from build123d import *

# Parameters (mm, degrees)
SKETCH1_R               = 43.5
SKETCH1_R_2             = 33.5
BOSS_EXTRUDE1_DEPTH     = 3
SKETCH3_R               = 2.025
CUT_EXTRUDE2_DEPTH      = 62.591395503
CIRPATTERN1_COUNT       = 12
CUT_EXTRUDE1_DEPTH      = 62.591395503
BOSS_EXTRUDE2_DEPTH     = 3
CUT_EXTRUDE_THIN1_DEPTH = 3
FILLET1_R               = 1.2
FILLET2_R               = 5
SKETCH6_R               = 2.525
CUT_EXTRUDE3_DEPTH      = 108.998410492
MIRROR4_OUTLINE_R       = 2.525
MIRROR4_DEPTH           = 3


# Read off the part's stored shape, not the designer's step: Mirror4
with BuildPart() as part:
    # Sketch1 → Boss-Extrude1 (new body)
    with BuildSketch(Plane(origin=(0, 0, 0), x_dir=(1, 0, 0), z_dir=(0, 1, 0))):
        with Locations(Location((0, 0, 0), (0, 0, 270))):
            Circle(SKETCH1_R)
        with Locations(Location((0, 0, 0), (0, 0, 270))):
            Circle(SKETCH1_R_2, mode=Mode.SUBTRACT)
    extrude(amount=BOSS_EXTRUDE1_DEPTH)

    # Sketch3 → Cut-Extrude2 (cut, symmetric)
    with BuildSketch(Plane(origin=(0, 3, 0), x_dir=(1, 0, 0), z_dir=(0, 1, 0))):
        with Locations(Location((-38, 0, 0), (0, 0, 270))):
            Circle(SKETCH3_R)
    cut_extrude2 = extrude(amount=CUT_EXTRUDE2_DEPTH, both=True, mode=Mode.SUBTRACT)

    # CirPattern1: Cut-Extrude2 ×12 about axis
    cirpattern1_axis = Axis((0, 0, 0), (0, 1, 0))
    for i in range(1, CIRPATTERN1_COUNT):
        add(cut_extrude2.rotate(cirpattern1_axis, i * 360 / CIRPATTERN1_COUNT), mode=Mode.SUBTRACT)

    # Sketch2 → Cut-Extrude1 (cut, symmetric)
    with BuildSketch(Plane(origin=(0, 3, 0), x_dir=(1, 0, 0), z_dir=(0, 1, 0))):
        with BuildLine():
            Line((0, 0), (43.5, 0))
            ThreePointArc((43.5, 0), (24.950574981, -35.633113927), (-14.877876235, -40.876629004))
            Line((-14.877876235, -40.876629004), (0, 0))
        make_face()
    cut_extrude1 = extrude(amount=CUT_EXTRUDE1_DEPTH, both=True, mode=Mode.SUBTRACT)

    # Mirror1: Cut-Extrude1 across plane
    add(cut_extrude1.mirror(Plane.XY), mode=Mode.SUBTRACT)

    # Sketch4 → Boss-Extrude2 (add)
    with BuildSketch(Plane(origin=(0, 0, 0), x_dir=(1, 0, 0), z_dir=(0, 1, 0))):
        with BuildLine():
            ThreePointArc((-33.322933276, -27.961261021), (-36.687527893, -23.372532963), (-39.424388736, -18.383894386))
            Line((-39.424388736, -18.383894386), (-57.550544477, -26.836259621))
            Line((-57.550544477, -26.836259621), (-76.583008005, -35.711243117))
            ThreePointArc((-76.583008005, -35.711243117), (-57.087372544, -62.29993496), (-28.900702111, -79.404026456))
            Line((-28.900702111, -79.404026456), (-21.718279101, -59.67048142))
            ThreePointArc((-21.718279101, -59.67048142), (-36.422103708, -52.016154812), (-48.643822138, -40.817013215))
            Line((-48.643822138, -40.817013215), (-33.322933276, -27.961261021))
        make_face()
    extrude(amount=BOSS_EXTRUDE2_DEPTH)

    # Sketch5 → Cut-Extrude-Thin1 (cut)
    with BuildSketch(Plane(origin=(0, 3, 0), x_dir=(1, 0, 0), z_dir=(0, 1, 0))):
        with BuildLine():
            ThreePointArc((-55.318354903, -43.219435568), (-42.735052316, -55.693404488), (-27.42932522, -64.619440712))
            Line((-27.42932522, -64.619440712), (-26.491570512, -62.410229064))
            ThreePointArc((-26.491570512, -62.410229064), (-41.274024887, -53.789356472), (-53.427129095, -41.741848027))
            Line((-53.427129095, -41.741848027), (-55.318354903, -43.219435568))
        make_face()
        with BuildLine():
            ThreePointArc((-62.804457062, -49.068219583), (-48.518285892, -63.230261221), (-31.141270941, -73.36423682))
            Line((-31.141270941, -73.36423682), (-30.203516232, -71.155025172))
            ThreePointArc((-30.203516232, -71.155025172), (-47.057258462, -61.326213205), (-60.913231254, -47.590632043))
            Line((-60.913231254, -47.590632043), (-62.804457062, -49.068219583))
        make_face()
    extrude(amount=-CUT_EXTRUDE_THIN1_DEPTH, mode=Mode.SUBTRACT)

    # Fillet1
    fillet1_edges = [part.edges().sort_by_distance(p)[0] for p in [
        (-55.318354903, 1.5, 43.219435568),
        (-62.804457062, 1.5, 49.068219583),
        (-53.427129095, 1.5, 41.741848027),
        (-60.913231254, 1.5, 47.590632043),
        (-26.491570512, 1.5, 62.410229064),
        (-30.203516232, 1.5, 71.155025172),
        (-27.42932522, 1.5, 64.619440712),
        (-31.141270941, 1.5, 73.36423682),
    ]]
    fillet(fillet1_edges, radius=FILLET1_R - 0.0001)  # a hair under: the kernel refuses the full size

    # Fillet2
    fillet2_edges = [part.edges().sort_by_distance(p)[0] for p in [
        (-14.877876235, 1.5, -40.876629004),
        (-11.457674801, 1.5, -31.479702796),
        (-11.457674801, 1.5, 31.479702796),
        (-14.877876235, 1.5, 40.876629004),
        (-39.424388736, 1.5, 18.383894386),
        (-76.583008005, 1.5, 35.711243117),
        (-28.900702111, 1.5, 79.404026456),
        (-21.718279101, 1.5, 59.67048142),
        (-33.322933276, 1.5, 27.961261021),
        (-48.643822138, 1.5, 40.817013215),
    ]]
    fillet(fillet2_edges, radius=FILLET2_R - 0.0001)  # a hair under: the kernel refuses the full size

    # Sketch6 → Cut-Extrude3 (cut, symmetric)
    with BuildSketch(Plane(origin=(0, 3, 0), x_dir=(1, 0, 0), z_dir=(0, 1, 0))):
        with Locations(Location((-58.287376448, -35.022589094, 0), (0, 0, 270))):
            Circle(SKETCH6_R)
        with Locations(Location((-66.859049455, -40.172969843, 0), (0, 0, 270))):
            Circle(SKETCH6_R)
    extrude(amount=CUT_EXTRUDE3_DEPTH, both=True, mode=Mode.SUBTRACT)

    # Mirror4 outline → Mirror4 (add)
    with BuildSketch(Plane(origin=(0, 0, 0), x_dir=(1, 0, 0), z_dir=(0, 1, 0))):
        with BuildLine():
            ThreePointArc((-33.837450466, 77.42917374), (-57.087372544, 62.29993496), (-74.185404229, 40.457085898))
            ThreePointArc((-74.185404229, 40.457085898), (-74.545675834, 36.50174496), (-71.908826648, 33.531636555))
            Line((-71.908826648, 33.531636555), (-43.721719229, 20.387772504))
            ThreePointArc((-43.721719229, 20.387772504), (-41.230877439, 17.806566879), (-41.109572338, 14.221570314))
            ThreePointArc((-41.109572338, 14.221570314), (-36.687527893, 23.372532963), (-30.262775922, 31.247630206))
            ThreePointArc((-30.262775922, 31.247630206), (-33.563151977, 29.842484947), (-36.955193962, 31.009089623))
            Line((-36.955193962, 31.009089623), (-44.649615181, 37.46547563))
            ThreePointArc((-44.649615181, 37.46547563), (-46.430731946, 41.073375084), (-44.977187998, 44.82524467))
            ThreePointArc((-44.977187998, 44.82524467), (-36.095854194, 52.243079063), (-26.015854641, 57.926033071))
            ThreePointArc((-26.015854641, 57.926033071), (-23.458659602, 60.540951414), (-23.365884028, 64.197238753))
            Line((-23.365884028, 64.197238753), (-27.136771358, 74.557666543))
            ThreePointArc((-27.136771358, 74.557666543), (-29.865761055, 77.443343725), (-33.837450466, 77.42917374))
        make_face()
        with Locations((-66.859049455, 40.172969843)):
            Circle(MIRROR4_OUTLINE_R, mode=Mode.SUBTRACT)
        with Locations((-58.287376448, 35.022589094)):
            Circle(MIRROR4_OUTLINE_R, mode=Mode.SUBTRACT)
        with BuildLine():
            ThreePointArc((-54.558346188, 44.174957399), (-42.735052316, 55.693404488), (-28.548993164, 64.132635914))
            ThreePointArc((-28.548993164, 64.132635914), (-27.6211406, 64.152839182), (-26.956370363, 63.505228894))
            ThreePointArc((-26.956370363, 63.505228894), (-26.944488545, 62.596515953), (-27.57295921, 61.940067165))
            ThreePointArc((-27.57295921, 61.940067165), (-41.274024887, 53.789356472), (-52.693103583, 42.664702445))
            ThreePointArc((-52.693103583, 42.664702445), (-53.489844598, 42.227547847), (-54.364518656, 42.474217018))
            ThreePointArc((-54.364518656, 42.474217018), (-54.818006961, 43.283949635), (-54.558346188, 44.174957399))
        make_face(mode=Mode.SUBTRACT)
        with BuildLine():
            ThreePointArc((-62.0470311, 50.02255423), (-48.518285891, 63.230261221), (-32.259123686, 72.879619504))
            ThreePointArc((-32.259123686, 72.879619504), (-31.332405, 72.898334407), (-30.668809601, 72.251187656))
            ThreePointArc((-30.668809601, 72.251187656), (-30.657391319, 71.341299876), (-31.287707164, 70.685001099))
            ThreePointArc((-31.287707164, 70.685001099), (-47.057258463, 61.326213205), (-60.178613602, 48.516228883))
            ThreePointArc((-60.178613602, 48.516228883), (-60.975687285, 48.077253152), (-61.851616121, 48.323778652))
            ThreePointArc((-61.851616121, 48.323778652), (-62.304960755, 49.13225649), (-62.0470311, 50.02255423))
        make_face(mode=Mode.SUBTRACT)
    extrude(amount=MIRROR4_DEPTH)


solid = part.part
CAD build for the part. Positions are in the model's coordinates, mm. A direction names the side the tool comes from. Round coordinates to 2 decimals unless told otherwise and drop trailing zeros. Order: outer loops, then holes, each group sorted by start corner. A loop starts at its lowest first (then second) coordinate and runs counter-clockwise, first axis right, second up. Notation, with made-up numbers: (15, 38.5) -> (26, 38.5) arc R29 cw to (26, 60.5) -> close; hole circle Ø7 at (33, 57). An arc over 180 degrees is marked (long way). Write item = value, one per line. Start each with the question number.
(1) Cut at A-A, the plane z = 0. List the corners of the cut face in (x, y) (3 decimals), then the cut area to 4 significant figures.
(2) Pin check, flat tips, straight feed: P1, Ø1.5, axis at x = -46, y = 0.5, coming from the -Z side; P2, Ø1, axis at y = 1, z = -41.5, coming from the -X side; P3, Ø2.5, axis at x = -32.91, z = 19, coming from the +Y side. Stop position of each tip, or through.
(3) Cut at B-B, the plane y = 1.75. State how many separate pieces and enclosed holes the cut face has, then the cut area to 3 significant figures.
(4) Cut at C-C, the plane z = -19. List the corners of the cut face in (x, y).
(5) Which spindle directions (+Z, -Z, +X, -X, +Y, -Y) get a long thin tool onto all of the face, cutting with end or side? Do faces 1 (the cylindrical face through (-41.21, 1.52, 17.76)), 2 (the cylindrical face through (-48.729, 1.521, 63.068)), 3 (the cylindrical face through (-36.23, 1.48, -52.15)). Say none if no direction does.
(6) Probe line 1 (Z direction, x = -28.5, y = 1.5); line 2 (X direction, y = 2.3, z = 0) (3 decimals); line 3 (Z direction, x = -60.5, y = 1.6). List the from-to ranges inside material, lowest first. Write a range as [from, to].
(7) Pull direction X, two halves, no side cores. Call faces 4 (the cylindrical face through (-36.3, 1.5, 1.1)), 5 (the flat face through (-41, 3, -6)), 6 (the cylindrical face through (-33.512, 1.521, 29.845)), 7 (the cylindrical face through (-29.81, 1.48, -77.42)): released by +X, released by -X, zero draft, split by the parting line, or undercut.
Model answer:
q1.outline = (-43.5, 0) -> (-40.025, 0) -> (-40.025, 3) -> (-43.5, 3) -> close; (-35.975, 0) -> (-33.5, 0) -> (-33.5, 3) -> (-35.975, 3) -> close
q1.area = 17.85 mm2
q2.P1 = -71.36
q2.P2 = -73.89
q2.P3 = through
q3.separate_pieces = 1
q3.enclosed_holes = 13
q3.area = 3,420 mm2
q4.outline = (-41.95, 0) -> (-34.93, 0) -> (-34.93, 3) -> (-41.95, 3) -> close; (-30.88, 0) -> (-27.59, 0) -> (-27.59, 3) -> (-30.88, 3) -> close
q5.face_1 = -X, +Y, -Y
q5.face_2 = +Y, -Y
q5.face_3 = +X, +Y, -Y
q6.line_1 = [-76.57, -64.15], [-61.52, -56.75], [-32.86, -17.61], [17.61, 32.86], [56.75, 61.52], [64.15, 76.57]
q6.line_2 = [-43.5, -40.025], [-35.975, -33.5]
q6.line_3 = [-58.99, -51.88], [-48.24, -36.24], [-33.81, -28.21], [28.21, 33.81], [36.24, 48.24], [51.88, 58.99]
q7.face_4 = undercut
q7.face_5 = zero draft
q7.face_6 = undercut
q7.face_7 = split by the parting line
